Check sheet for the drawn part. Datum: minimum x, y, z corner. Units: mm. Round coordinates to 2 decimals unless told otherwise and drop trailing zeros. Write each loop counter-clockwise with the first axis right and the second up, starting at its lowest first coordinate (ties: lowest second). Pieces come first, ordered by that corner, then holes. Notation, with made-up numbers: (-18, 77.5) - (1, 77.5) arc R22 ccw to (1, 113.5) - close; hole circle Ø8 at (18, 38.5). An arc over 180 degrees is marked (long way). Answer as a JSON object with one key per item and string values.
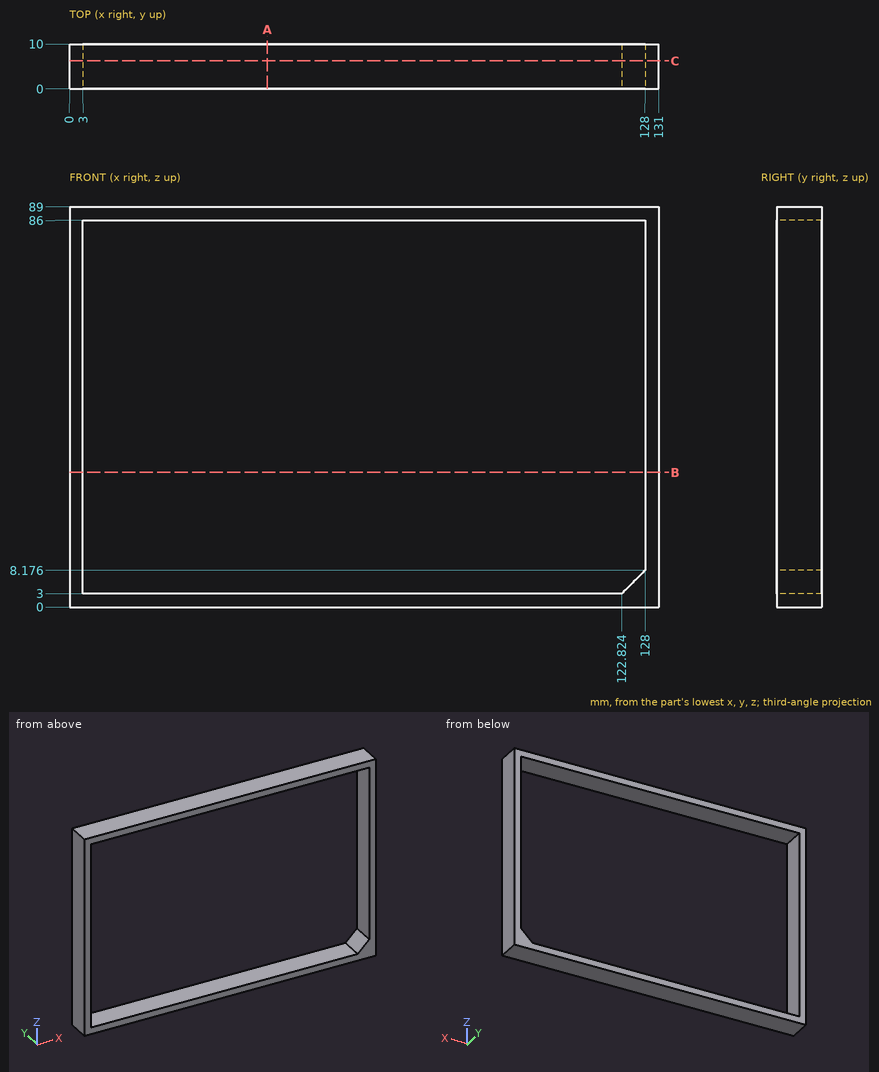
1. Cross-section at A-A (x = 44). Record the boundary of the cut face in (y, z), plus the area to 3 significant figures.
Completed:
{"outline": "(0, 0) - (10, 0) - (10, 3) - (0, 3) - close; (0, 86) - (10, 86) - (10, 89) - (0, 89) - close", "area": "60.0 mm^2"}
2. Cross-section at C-C (y = 6.25). Record the boundary of the cut face in (x, z).
Completed:
{"outline": "(0, 0) - (131, 0) - (131, 89) - (0, 89) - close; hole (3, 3) - (122.82, 3) - (128, 8.18) - (128, 86) - (3, 86) - close"}
3. Go/stop test with a flat-tipped pin: pin 1 (6 mm diameter, centred on x = 72, y = 8, fed in from -Z). Record where the tip stops, or that it passes through.
Completed:
{"pin 1": "stops at z = 0"}
4. Cross-section at B-B (z = 30). Record the boundary of the cut face in (x, y), plus the area to 3 significant figures.
Completed:
{"outline": "(0, 0) - (3, 0) - (3, 10) - (0, 10) - close; (128, 0) - (131, 0) - (131, 10) - (128, 10) - close", "area": "60.0 mm^2"}
5. Material ranges on probe 1 along Z at (x, y) = (102.5, 5); probe 2 along X at (y, z) = (7.75, 27), recorded low to high. Write a range as from..to.
Completed:
{"probe 1": "z = 0..3, 86..89", "probe 2": "x = 0..3, 128..131"}
